The listing builds one solid part. Answer for the finished solid, in the listing's coordinates (mm). A direction names the side the tool comes from. Give positions to 0.01 mm unless a question says otherwise; leave off trailing zeros. Order: outer loops, then holes, each group sorted by start corner. A loop starts at its lowest first (then second) coordinate and runs counter-clockwise, first axis right, second up.
```python
from build123d import *

# Parameters (mm, degrees)
F0_W     = 493.776
F0_H     = 457.2
F0_W_2   = 19.812
F0_H_2   = 241.3
F1_DEPTH = 5.08
F2_R     = 1.016
F3_DEPTH = 5.081
F5_DEPTH = 5.081
F6_DEPTH = 5.08


# Not quite as in the source:
# - a feature names something its author has since deleted; it is built from what else it names


with BuildPart() as f1:
    # F0 (on Front) → F1 (new body)
    with BuildSketch(Plane.XZ):
        with Locations((246.888, 228.6)):
            Rectangle(F0_W, F0_H)
        with Locations((188.9506, 228.6)):
            Rectangle(F0_W_2, F0_H_2, mode=Mode.SUBTRACT)
        with Locations((304.8254, 228.6)):
            Rectangle(F0_W_2, F0_H_2, mode=Mode.SUBTRACT)
    extrude(amount=F1_DEPTH)

    # F2 (on face) → F3 (cut, through all)
    with BuildSketch(Plane.XZ.offset(5.08)):
        with Locations((56.388, 381)):
            Circle(F2_R)
        with Locations((56.388, 76.2)):
            Circle(F2_R)
        with Locations((437.388, 76.2)):
            Circle(F2_R)
        with Locations((437.388, 381)):
            Circle(F2_R)
    extrude(amount=-F3_DEPTH, mode=Mode.SUBTRACT)

    # F4 (on face) → F5 (cut, through all)
    with BuildSketch(Plane.XZ.offset(5.08)):
        with BuildLine():
            Line((80.2894, 349.25), (54.8894, 349.25))
            ThreePointArc((54.8894, 349.25), (18.9683755157, 334.3710244843), (4.0894, 298.45))
            Line((4.0894, 298.45), (4.0894, 158.75))
            ThreePointArc((4.0894, 158.75), (18.9683755157, 122.8289755157), (54.8894, 107.95))
            Line((54.8894, 107.95), (80.2894, 107.95))
            ThreePointArc((80.2894, 107.95), (116.2104244843, 122.8289755157), (131.0894, 158.75))
            Line((131.0894, 158.75), (131.0894, 298.45))
            ThreePointArc((131.0894, 298.45), (116.2104244843, 334.3710244843), (80.2894, 349.25))
        make_face()
        with BuildLine():
            Line((438.8866, 349.25), (413.4866, 349.25))
            ThreePointArc((413.4866, 349.25), (377.5655755157, 334.3710244843), (362.6866, 298.45))
            Line((362.6866, 298.45), (362.6866, 158.75))
            ThreePointArc((362.6866, 158.75), (377.5655755157, 122.8289755157), (413.4866, 107.95))
            Line((413.4866, 107.95), (438.8866, 107.95))
            ThreePointArc((438.8866, 107.95), (474.8076244843, 122.8289755157), (489.6866, 158.75))
            Line((489.6866, 158.75), (489.6866, 298.45))
            ThreePointArc((489.6866, 298.45), (474.8076244843, 334.3710244843), (438.8866, 349.25))
        make_face()
    extrude(amount=-F5_DEPTH, mode=Mode.SUBTRACT)

    # F2 (on face) → F6 (cut, through all)
    with BuildSketch(Plane.XZ.offset(5.08)):
        with Locations((246.888, 304.8)):
            Circle(F2_R)
        with Locations((246.888, 152.4)):
            Circle(F2_R)
    extrude(amount=-F6_DEPTH, mode=Mode.SUBTRACT)


solid = f1.part
```
1) Straight lines are drawn through the part: probe 1 along X at (y, z) = (-4.05, 231.5); probe 2 along Z at (x, y) = (420, -4.8); probe 3 along X at (y, z) = (-1.7, 304.8). For each, find the intervals that lie inside material, in ascending order.
Geometry says:
probe 1: x = 0 to 4.09, 131.09 to 179.04, 198.86 to 294.92, 314.73 to 362.69, 489.69 to 493.78
probe 2: z = 0 to 107.95, 349.25 to 457.2
probe 3: x = 0 to 4.49, 130.69 to 179.04, 198.86 to 245.87, 247.9 to 294.92, 314.73 to 363.09, 489.29 to 493.78
2) Find section A-A (x = 425). Write down the section's boundary in (y, z).
Geometry says:
outline: (-5.08, 0) - (0, 0) - (0, 107.95) - (-5.08, 107.95) - close; (-5.08, 349.25) - (0, 349.25) - (0, 457.2) - (-5.08, 457.2) - close
3) Find section C-C (y = -1.55). Count the separate pieces of the cut face and the enclosed holes in it, then the cut area to 3 significant figures.
Geometry says:
separate pieces: 1
enclosed holes: 10
area: 159,000 mm2
4) For a pull along Z with two mould halves and no side action, classify faces 1 (the flat face through (243, 0, 232)), 2 (the cylindrical face through (116.603, -2.576, 333.974)) as +Z half, -Z half, draft (parallel to the pull), parting line (faces both ways), or undercut.
Geometry says:
face 1: draft
face 2: undercut
5) Find section B-B (z = 211.5). Write down the section's boundary in (x, y), then the cut area to 3 significant figures.
Geometry says:
outline: (0, -5.08) - (4.09, -5.08) - (4.09, 0) - (0, 0) - close; (131.09, -5.08) - (179.04, -5.08) - (179.04, 0) - (131.09, 0) - close; (198.86, -5.08) - (294.92, -5.08) - (294.92, 0) - (198.86, 0) - close; (314.73, -5.08) - (362.69, -5.08) - (362.69, 0) - (314.73, 0) - close; (489.69, -5.08) - (493.78, -5.08) - (493.78, 0) - (489.69, 0) - close
area: 1,020 mm2
6) Find section D-D (x = 30). Write down the section's boundary in (y, z).
Geometry says:
outline: (-5.08, 0) - (0, 0) - (0, 114.47) - (-5.08, 114.47) - close; (-5.08, 342.73) - (0, 342.73) - (0, 457.2) - (-5.08, 457.2) - close
7) A tool of negligible diameter and unlimited length cuts with its end or side. For faces 3 (the flat face through (243, -5.08, 232)), 4 (the cylindrical face through (18.6, -2.6, 123.2)), from which of +Z, -Z, +X, -X, +Y, -Y can it reach the whole face along a straight path? Write none if from no direction.
Geometry says:
face 3: +Z, -Z, +X, -X, -Y
face 4: +Y, -Y
